Here's how the part is built. I have some questions about the finished solid (model axes, mm). Face numbers are marked on the shaded views. A direction names the side the tool comes from. Give positions to 0.01 mm unless a question says otherwise; leave off trailing zeros. Write each loop counter-clockwise with the first axis right and the second up, starting at its lowest first coordinate (ties: lowest second). Pieces come first, ordered by that corner, then holes. Notation, with made-up numbers: (-9, 61.25) - (20, 61.25) arc R13 ccw to (20, 70.25) - close; hole circle Ø10 at (3, -36.5). An arc over 180 degrees is marked (long way). Write each question's results on one line, items separated by ' | '. Start each with the question number.
Item 1: Suppose I cut it at C-C on x = 5.5. List the corners of the cut face in (y, z) for me.
Item 2: Suppose I cut it at D-D on z = 135.5. List the corners of the cut face in (x, y) for me, then the cut area to 3 significant figures.
Item 3: We'd pull the mould along Z, two halves only. Please class the marked faces 1, 2 and 3: +Z half, -Z half, draft (parallel to the pull), parting line (faces both ways), or undercut.
Item 4: Please list where these lines run through material, in increasing order: line 1 along Y through (x, z) = (36, 143.5); line 2 along X through (y, z) = (-7.5, 33.5); line 3 along Z through (x, y) = (19.5, 2.5).
Item 5: Which directions (+Z, -Z, +X, -X, +Y, -Y) give clear straight access to the entire face, cutting with the end or side of a thin tool? Please do the marked faces 4, 5 and 6.
Item 6: Suppose I cut it at B-B on y = -5.1. List the corners of the cut face in (x, z) for me.
Item 7: Will these pins go through, and if not, where does the flat tip stop? P1, Ø4, axis at x = 28, z = 91.5, coming from the +Y side; P2, Ø8, axis at x = 12.5, y = -33, coming from the -Z side; P3, Ø1.5, axis at x = 22.5, z = -1, coming from the -Y side.
Autodesk Inventor part; units mm, degrees
ref_plane "YZ Plane" through (0, 0, 0) normal (1, 0, 0) x (0, 1, 0)
ref_plane "XZ Plane" through (0, 0, 0) normal (0, 1, 0) x (-1, 0, 0)
ref_plane "XY Plane" through (0, 0, 0) normal (0, 0, 1) x (1, 0, 0)
sketch "Sketch1" plane through (0, 0, 0) normal (0, 0, 1) x (1, 0, 0)
  line L0 (0, 0) -> (74, 0)
  line L1 (74, 0) -> (74, -7.6)
  line L2 (74, -7.6) -> (0, -7.6)
  line L3 (0, -7.6) -> (0, 0)
  line L4 (0.9, 13.2) -> (73.1, 13.2)
  line L5 (73.1, 13.2) -> (73.1, 12)
  line L6 (73.1, 12) -> (0.9, 12)
  line L7 (0.9, 12) -> (0.9, 13.2)
  line L8 (-3, 16.2) -> (77, 16.2)
  line L9 (77, 16.2) -> (77, -10.6)
  line L10 (77, -10.6) -> (-3, -10.6)
  line L11 (-3, -10.6) -> (-3, 16.2)
  dimension "d0" = 74
  dimension "d1" = 7.6
  dimension "d2" = 1.2
  dimension "d3" = 12
  dimension "d4" = 72.2
  dimension "d5" = 0.9
  dimension "d6" = 3
  dimension "d7" = 3
  dimension "d8" = 3
  dimension "d9" = 3
extrude "Extrusion1" add sketch "Sketch1" along normal blind 151.5
sketch "Sketch2" plane through (-3, 16.2, 0) normal (0, 1, 0) x (1, 0, 0)
  line L0 (77, -12.1) -> (3, -12.1)
  line L1 (3, -12.1) -> (3, -137.5)
  line L2 (3, -137.5) -> (77, -137.5)
  line L3 (77, -137.5) -> (77, -12.1)
  line L4 (80, 0) -> (80, -151.5)
  line L5 (0, 0) -> (0, -151.5)
  line L6 (80, 0) -> (0, 0)
  line L7 (80, -151.5) -> (0, -151.5)
  point P0 (3, 0)
  dimension "d12" = 3
  dimension "d14" = 12.1
  dimension "d15" = 14
  dimension "d23" = 3
extrude "Extrusion2" cut sketch "Sketch2" against normal up to surface (23.8 mm away) contours L3 L2 L1 L0
sketch "Sketch3" plane through (-3, 16.2, 0) normal (0, 1, 0) x (1, 0, 0)
  line L0 (80, 0) -> (80, -151.5)
  line L1 (0, 0) -> (0, -151.5)
  line L2 (80, -0.75) -> (0, -0.75)
  line L3 (0, -0.75) -> (0, -150.75)
  line L4 (0, -150.75) -> (80, -150.75)
  line L5 (80, -150.75) -> (80, -0.75)
  line L6 (80, -151.5) -> (0, -151.5)
  line L7 (80, 0) -> (0, 0)
  line L8 (80, 0) -> (0, 0)
  line L9 (0, 0) -> (0, -151.5)
  line L10 (0, -151.5) -> (80, -151.5)
  line L11 (80, -151.5) -> (80, 0)
  point P0 (3, 0)
  point P1 (0, -0.75)
  dimension "d18" = 150
  dimension "d19" = 151.5
  dimension "d20" = 0.75
extrude "Extrusion3" add sketch "Sketch3" against normal up to surface (4.2 mm away) contours L0 L2 L1 L7 | L0 L6 L1 L4
sketch "Sketch4" plane through (0, 0, 0) normal (0, 0, -1) x (-1, 0, 0)
  line L0 (-77, -10.6) -> (-77, 16.2)
  line L1 (3, 16.2) -> (3, -10.6)
  line L2 (-77, -10.6) -> (3, -10.6)
  line L3 (3, -10.6) -> (3, 16.2)
  line L4 (3, 16.2) -> (-77, 16.2)
  line L5 (-77, 16.2) -> (-77, -10.6)
  point P0 (0, 0)
extrude "Extrusion4" add sketch "Sketch4" along normal blind 3
sketch "Sketch5" plane through (0, 0, 151.5) normal (0, 0, 1) x (1, 0, 0)
  line L0 (-3, 16.2) -> (77, 16.2)
  line L1 (77, -10.6) -> (-3, -10.6)
  line L2 (77, 16.2) -> (-3, 16.2)
  line L3 (-3, 16.2) -> (-3, -10.6)
  line L4 (-3, -10.6) -> (77, -10.6)
  line L5 (77, -10.6) -> (77, 16.2)
  line L6 (43.5, -0.4) -> (30.5, -0.4)
  line L7 (30.5, -0.4) -> (30.5, -7.2)
  line L8 (30.5, -7.2) -> (43.5, -7.2)
  line L9 (43.5, -7.2) -> (43.5, -0.4)
  line L10 (74, -7.6) -> (0, -7.6)
  line L11 (74, 0) -> (74, -7.6)
  point P0 (0, 0)
  dimension "d26" = 6.8
  dimension "d27" = 13
  dimension "d28" = 0.4
  dimension "d29" = 30.5
extrude "Extrusion5" add sketch "Sketch5" along normal blind 3
sketch "Sketch6" plane through (-3, -10.6, -3) normal (0, -1, 0) x (1, 0, 0)
  line L0 (48, 14.3) -> (32, 14.3)
  line L1 (32, 14.3) -> (32, 32)
  line L2 (32, 32) -> (48, 32)
  line L3 (48, 32) -> (48, 14.3)
  line L4 (77, 3) -> (3, 3)
  line L5 (80, 157.5) -> (80, 0)
  dimension "d32" = 11.3
  dimension "d33" = 16
  dimension "d34" = 17.7
  dimension "d35" = 32
extrude "Extrusion6" cut sketch "Sketch6" against normal up to surface (3 mm away)
sketch "Sketch7" plane through (-3, 16.2, -3) normal (0, 1, 0) x (1, 0, 0)
  line L0 (3, -15.1) -> (77, -15.1)
  line L1 (77, -140.5) -> (3, -140.5)
  line L2 (74.6, -15.1) -> (5.4, -15.1)
  line L3 (5.4, -15.1) -> (5.4, -140.5)
  line L4 (5.4, -140.5) -> (74.6, -140.5)
  line L5 (74.6, -140.5) -> (74.6, -15.1)
  line L6 (77, -15.1) -> (77, -140.5)
  line L7 (3, -140.5) -> (3, -15.1)
  line L8 (77, -3) -> (77, -15.1)
  line L9 (77, -15.1) -> (3, -15.1)
  line L10 (3, -15.1) -> (3, -140.5)
  line L11 (3, -140.5) -> (77, -140.5)
  line L12 (77, -140.5) -> (77, -15.1)
  point P0 (3, -3)
  point P1 (5.4, -15.1)
  dimension "d38" = 2.4
  dimension "d39" = 2.4
extrude "Extrusion7" add sketch "Sketch7" against normal up to surface (3 mm away) contours L0 L3 L1 L7 | L0 L6 L1 L5
sketch "Sketch8" plane through (0, 0, -3) normal (0, 0, -1) x (-1, 0, 0)
  line L0 (-74, -7.6) -> (0, -7.6)
  line L1 (-18.5, -7.6) -> (-28.5, -7.6)
  line L2 (-31, -5.1) -> (-31, -5.1)
  line L3 (-28.5, -2.6) -> (-18.5, -2.6)
  line L4 (-16, -5.1) -> (-16, -5.1)
  line L5 (0, -7.6) -> (0, 0)
  line L6 (0, 0) -> (-74, 0)
  arc A0 (-31, -5.1) -> (-28.5, -7.6) centre (-28.5, -5.1) ccw
  arc A1 (-28.5, -2.6) -> (-31, -5.1) centre (-28.5, -5.1) ccw
  arc A2 (-18.5, -7.6) -> (-16, -5.1) centre (-18.5, -5.1) ccw
  arc A3 (-16, -5.1) -> (-18.5, -2.6) centre (-18.5, -5.1) ccw
  point P0 (-16, -7.6)
  point P1 (-31, -2.6)
  point P2 (-31, -7.6)
  point P3 (-16, -2.6)
  dimension "d42" = 15
  dimension "d43" = 16
  dimension "d44" = 2.6
  dimension "d45" = 5
  dimension "d46" = 2.5
extrude "Extrusion8" cut sketch "Sketch8" against normal up to surface (3 mm away)
sketch "Sketch9" plane through (0, 0, 12.1) normal (0, 0, 1) x (1, 0, 0)
  line L0 (0.9, 12) -> (0.9, 13.2)
  line L1 (0.9, 12) -> (0, 12)
  line L2 (0, 13.2) -> (0, 0)
  line L3 (0, 12) -> (1.9, 12)
  line L4 (1.9, 12) -> (1.9, 10.5)
  line L5 (1.9, 10.5) -> (0, 10.5)
  line L6 (0, 10.5) -> (0, 12)
  line L7 (0.9, 13.2) -> (0, 13.2)
  line L8 (0, 13.2) -> (0, 12)
  line L9 (0, 12) -> (0.9, 12)
  line L10 (0.9, 12) -> (0.9, 13.2)
  line L11 (73.1, 12) -> (73.1, 13.2)
  line L12 (73.1, 12) -> (74, 12)
  line L13 (74, 13.2) -> (74, 0)
  line L14 (74, 12) -> (72.1, 12)
  line L15 (72.1, 12) -> (72.1, 10.5)
  line L16 (72.1, 10.5) -> (74, 10.5)
  line L17 (74, 10.5) -> (74, 12)
  line L18 (74, 13.2) -> (73.1, 13.2)
  line L19 (73.1, 12) -> (74, 12)
  line L20 (74, 12) -> (74, 13.2)
  line L21 (74, 13.2) -> (73.1, 13.2)
  line L22 (73.1, 13.2) -> (73.1, 12)
  point P0 (0, 10.5)
  point P1 (73.1, 12)
  dimension "d49" = 1
  dimension "d50" = 1.5
  dimension "d52" = 1.5
  dimension "d53" = 1
extrude "Extrusion9" add sketch "Sketch9" along normal up to surface (125.4 mm away)
sketch "Sketch10" plane through (-3, -10.6, -3) normal (0, -1, 0) x (1, 0, 0)
  line L0 (20, 98.75) -> (-20, 98.75)
  line L1 (-20, 98.75) -> (-20, 58.75)
  line L2 (-20, 58.75) -> (20, 58.75)
  line L3 (20, 58.75) -> (20, 98.75)
  line L4 (80, 0) -> (0, 0)
  line L5 (0, 0) -> (0, 157.5)
  point P0 (3, 3)
  dimension "d56" = 40
  dimension "d57" = 40
  dimension "d58" = 58.75
  dimension "d59" = 20
extrude "Extrusion10" cut sketch "Sketch10" against normal blind 13.4
chamfer "Chamfer1" distance 3 angle 45 1 edges at (17, -7.6, 75.75)
sketch "Sketch12" plane through (-3, -10.6, 55.75) normal (0, 0, 1) x (1, 0, 0)
  line L0 (-17.0576, 7.8863) -> (11.2267, -20.3979)
  line L1 (11.2267, -20.3979) -> (4.1557, -27.469)
  line L2 (4.1557, -27.469) -> (-24.1286, 0.8153)
  line L3 (-24.1286, 0.8153) -> (-17.0576, 7.8863)
  line L4 (80, 0) -> (0, 0)
  line L5 (0, 13.4) -> (3, 16.4)
  line L6 (3, 16.4) -> (-17.0576, 7.8863)
  line L7 (23, 3) -> (20, 0)
  line L8 (23, 3) -> (11.2267, -20.3979)
  line L9 (23, 3) -> (3, 16.4)
  point P0 (3, 10.6)
  point P1 (21.4905, 0)
  dimension "d65" = 90
  dimension "d66" = 90
  dimension "d67" = 45
  dimension "d68" = 10
  dimension "d69" = 40
extrude "Extrusion11" cut sketch "Sketch12" along normal up to surface (40 mm away) contours L6 L9 L7 L4 L8 L0 | L4 L7 L8
sketch "Sketch13" plane through (-3, -10.6, 55.75) normal (0, 0, 1) x (1, 0, 0)
  line L0 (-17.0576, 7.8863) -> (11.2267, -20.3979)
  line L1 (11.2267, -20.3979) -> (4.1557, -27.469)
  line L2 (4.1557, -27.469) -> (-24.1286, 0.8153)
  line L3 (-24.1286, 0.8153) -> (-17.0576, 7.8863)
  line L4 (3, 16.4) -> (-17.0576, 7.8863)
  line L5 (23, 3) -> (11.2267, -20.3979)
  line L6 (23, 3) -> (3, 16.4) construction
  line L7 (-18.1567, 11.0298) -> (-26.2499, 2.9366)
  line L8 (-28.3713, 0.8153) -> (4.1557, -31.7116) construction
  line L9 (6.277, -29.5903) -> (18.682, -17.1853)
  line L10 (-24.1286, 0.8153) -> (-26.2499, 2.9366)
  line L11 (-26.2499, 2.9366) -> (6.277, -29.5903)
  line L12 (-1.8502, 17.6004) -> (-8.6324, 14.7216)
  line L13 (-1.8502, 17.6004) -> (-22.9463, 8.6459)
  line L14 (-9.9896, 14.1455) -> (3.638, 19.9299)
  line L15 (0, 0) -> (0, 26.8)
  line L16 (0, 15.1266) -> (0, 18.3857)
  line L17 (0, 0) -> (0, 15.1266)
  line L18 (23.2213, -3.2345) -> (18.7952, -12.0308)
  line L19 (23.2213, -3.2345) -> (9.1734, -31.1531)
  line L20 (17.9281, -13.7542) -> (27.2379, 4.7479)
  line L21 (80, 0) -> (0, 0)
  line L22 (24.8488, 0) -> (21.4905, 0)
  point P0 (3, 10.6)
  point P1 (4, 11.6)
  point P2 (0, 18.3857)
  point P3 (-8.6324, 14.7216)
  point P4 (-18.7665, 10.42)
  point P5 (13.6895, -22.1778)
  point P6 (23.2213, -3.2345)
  dimension "d72" = 90
  dimension "d73" = 90
  dimension "d74" = 10
  dimension "d75" = 40
  dimension "d76" = 3
  dimension "d77" = 3
  dimension "d78" = 3
  dimension "d79" = 3
  dimension "d80" = 3
extrude "Extrusion12" add sketch "Sketch13" along normal up to surface (40 mm away) contours L3 L10 L7 L13 L12 L14 L15 L4 | L5 L21 L20 L18 L19 L9 L11 L1
properties part number "left"
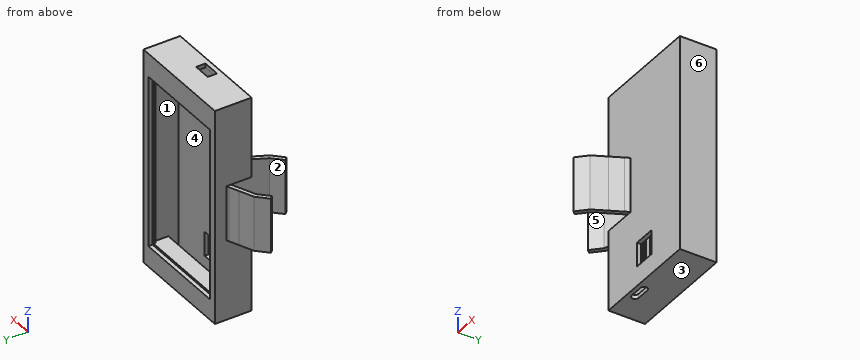
Checked values:
1) outline: (-37.97, 55.75) - (-33.72, 55.75) - (-33.72, 95.75) - (-37.97, 95.75) - close; (-10.6, -3) - (16.2, -3) - (16.2, 12.1) - (13.2, 12.1) - (13.2, 0.75) - (12, 0.75) - (12, 12.1) - (0, 12.1) - (0, 0) - (-7.6, 0) - (-7.6, 55.75) - (-10.6, 55.75) - close; (-10.6, 95.75) - (-7.6, 95.75) - (-7.6, 151.5) - (0, 151.5) - (0, 137.5) - (12, 137.5) - (12, 150.75) - (13.2, 150.75) - (13.2, 137.5) - (16.2, 137.5) - (16.2, 154.5) - (-10.6, 154.5) - close
2) outline: (-3, -10.6) - (77, -10.6) - (77, 16.2) - (71.6, 16.2) - (71.6, 13.2) - (73.1, 13.2) - (73.1, 12) - (72.1, 12) - (72.1, 10.5) - (74, 10.5) - (74, -7.6) - (0, -7.6) - (0, 10.5) - (1.9, 10.5) - (1.9, 12) - (0.9, 12) - (0.9, 13.2) - (2.4, 13.2) - (2.4, 16.2) - (-3, 16.2) - close | area: 405 mm^2
3) face 1: undercut | face 2: draft | face 3: -Z half
4) line 1: y = -10.6 to -7.6, 0 to 12, 13.2 to 16.2 | line 2: x = -3 to 0, 74 to 77 | line 3: z = -3 to 12.1, 137.5 to 154.5
5) face 4: none | face 5: +Z, -Z, -Y | face 6: +Z, -Z, +X, +Y, -Y
6) outline: (-26.69, 55.75) - (-22.44, 55.75) - (-22.44, 95.75) - (-26.69, 95.75) - close; (-3, -3) - (16, -3) - (16, 0) - (0, 0) - (0, 55.75) - (-3, 55.75) - close; (-3, 95.75) - (0, 95.75) - (0, 151.5) - (30.5, 151.5) - (30.5, 154.5) - (-3, 154.5) - close; (31, -3) - (77, -3) - (77, 154.5) - (43.5, 154.5) - (43.5, 151.5) - (74, 151.5) - (74, 0) - (31, 0) - close
7) P1: stops at y = -7.6 | P2: stops at z = 55.75 | P3: stops at y = -10.6
